```python
from build123d import *

# Parameters (mm, degrees)
SKETCH1_R               = 20
BOSS_EXTRUDE1_DEPTH     = 4
SKETCH2_R               = 1.25
CUT_EXTRUDE1_DEPTH      = 29.565713714
CAVITY1_START           = 2.8
CAVITY1_OUTLINE_R       = 0.675
CAVITY1_OUTLINE_R_2     = 0.6
CAVITY1_OUTLINE_R_3     = 2.5
CAVITY1_DEPTH           = 1.2
CAVITY1_START_2         = 3.4
CAVITY1_2_OUTLINE_R     = 2.5
CAVITY1_2_OUTLINE_R_2   = 1.25
CAVITY1_2_DEPTH         = 0.6
CUT_EXTRUDE2_START      = -2
CUT_EXTRUDE2_DEPTH      = 2
CUT_EXTRUDE3_START      = -1.2
CUT_EXTRUDE3_DEPTH      = 1.2
CUT_EXTRUDE4_DEPTH      = 1.2
SKETCH6_R               = 1.25
CUT_EXTRUDE5_DEPTH      = 29.565713714
CIRPATTERN1_COUNT       = 4
CUT_EXTRUDE6_DEPTH      = 29.422526278
CUT_EXTRUDE6_DEPTH_BACK = 2.4
SKETCH7_R               = 3.8
SKETCH8_R               = 20
SKETCH8_R_2             = 2.5
SKETCH8_R_3             = 1.25
BOSS_EXTRUDE2_DEPTH     = 3.5
CUT_EXTRUDE7_DEPTH      = 2.5
SKETCH10_R              = 2.5
SKETCH10_R_2            = 1.25
BOSS_EXTRUDE4_DEPTH     = 0.8
SKETCH11_R              = 2.5
SKETCH11_R_2            = 1.25
BOSS_EXTRUDE5_DEPTH     = 1.2
SKETCH12_R              = 3.8
CUT_EXTRUDE8_DEPTH      = 0.8


# Read off the part's stored shape, not the designer's step: Cavity1
with BuildPart() as part:
    # Sketch1 → Boss-Extrude1 (new body)
    with BuildSketch(Plane.XY):
        Circle(SKETCH1_R)
    extrude(amount=BOSS_EXTRUDE1_DEPTH)

    # Sketch2 → Cut-Extrude1 (cut, through all)
    with BuildSketch(Plane.XY.offset(4)):
        Circle(SKETCH2_R)
    extrude(amount=-CUT_EXTRUDE1_DEPTH, mode=Mode.SUBTRACT)

    # Cavity1 outline → Cavity1 (cut)
    with BuildSketch(Plane.XY.offset(CAVITY1_START)):
        with BuildLine():
            ThreePointArc((2.993325909, 2), (2.762479071, 2.308399745), (2.5, 2.590366769))
            Line((2.5, 2.590366769), (2.5, 3.6))
            Line((2.5, 3.6), (2, 15.6))
            ThreePointArc((2, 15.6), (0, 17.6), (-2, 15.6))
            Line((-2, 15.6), (-2.5, 3.6))
            Line((-2.5, 3.6), (-2.5, 2.590366769))
            ThreePointArc((-2.5, 2.590366769), (-2.762479071, 2.308399745), (-2.993325909, 2))
            Line((-2.993325909, 2), (-6.6, 2))
            ThreePointArc((-6.6, 2), (-8.6, 0), (-6.6, -2))
            Line((-6.6, -2), (-2.993325909, -2))
            ThreePointArc((-2.993325909, -2), (-2.762479071, -2.308399745), (-2.5, -2.590366769))
            Line((-2.5, -2.590366769), (-2.5, -3.6))
            Line((-2.5, -3.6), (-2, -15.6))
            ThreePointArc((-2, -15.6), (0, -17.6), (2, -15.6))
            Line((2, -15.6), (2.5, -3.6))
            Line((2.5, -3.6), (2.5, -2.590366769))
            ThreePointArc((2.5, -2.590366769), (2.762479071, -2.308399745), (2.993325909, -2))
            Line((2.993325909, -2), (6.6, -2))
            ThreePointArc((6.6, -2), (8.6, 0), (6.6, 2))
            Line((6.6, 2), (2.993325909, 2))
        make_face()
        with Locations((0, -15.6)):
            Circle(CAVITY1_OUTLINE_R, mode=Mode.SUBTRACT)
        with Locations((0, -13.4)):
            Circle(CAVITY1_OUTLINE_R, mode=Mode.SUBTRACT)
        with Locations((0, -11.2)):
            Circle(CAVITY1_OUTLINE_R, mode=Mode.SUBTRACT)
        with Locations((0, -9)):
            Circle(CAVITY1_OUTLINE_R, mode=Mode.SUBTRACT)
        with Locations((0, -6.8)):
            Circle(CAVITY1_OUTLINE_R, mode=Mode.SUBTRACT)
        with Locations((0, -4.6)):
            Circle(CAVITY1_OUTLINE_R, mode=Mode.SUBTRACT)
        with Locations((-6.6, 0)):
            Circle(CAVITY1_OUTLINE_R_2, mode=Mode.SUBTRACT)
        with Locations((-4.6, 0)):
            Circle(CAVITY1_OUTLINE_R_2, mode=Mode.SUBTRACT)
        Circle(CAVITY1_OUTLINE_R_3, mode=Mode.SUBTRACT)
        with Locations((0, 4.6)):
            Circle(CAVITY1_OUTLINE_R, mode=Mode.SUBTRACT)
        with Locations((0, 6.8)):
            Circle(CAVITY1_OUTLINE_R, mode=Mode.SUBTRACT)
        with Locations((4.6, 0)):
            Circle(CAVITY1_OUTLINE_R_2, mode=Mode.SUBTRACT)
        with Locations((6.6, 0)):
            Circle(CAVITY1_OUTLINE_R_2, mode=Mode.SUBTRACT)
        with Locations((0, 9)):
            Circle(CAVITY1_OUTLINE_R, mode=Mode.SUBTRACT)
        with Locations((0, 11.2)):
            Circle(CAVITY1_OUTLINE_R, mode=Mode.SUBTRACT)
        with Locations((0, 13.4)):
            Circle(CAVITY1_OUTLINE_R, mode=Mode.SUBTRACT)
        with Locations((0, 15.6)):
            Circle(CAVITY1_OUTLINE_R, mode=Mode.SUBTRACT)
    extrude(amount=CAVITY1_DEPTH, mode=Mode.SUBTRACT)

    # Cavity1 2 outline → Cavity1 2 (cut)
    with BuildSketch(Plane.XY.offset(CAVITY1_START_2)):
        Circle(CAVITY1_2_OUTLINE_R)
        Circle(CAVITY1_2_OUTLINE_R_2, mode=Mode.SUBTRACT)
    extrude(amount=CAVITY1_2_DEPTH, mode=Mode.SUBTRACT)

    # Sketch3 → Cut-Extrude2 (cut)
    with BuildSketch(Plane.XY.offset(3.4).offset(CUT_EXTRUDE2_START)):
        with BuildLine():
            ThreePointArc((-2.5, 0), (0, -2.5), (2.5, 0))
            ThreePointArc((2.5, 0), (0, 2.5), (-2.5, 0))
        make_face()
    extrude(amount=CUT_EXTRUDE2_DEPTH, mode=Mode.SUBTRACT)

    # Sketch4 → Cut-Extrude3 (cut)
    with BuildSketch(Plane.XY.offset(4).offset(CUT_EXTRUDE3_START)):
        with BuildLine():
            Line((-6.6, -2), (-2.993325909, -2))
            ThreePointArc((-2.993325909, -2), (-2.762479071, -2.308399745), (-2.5, -2.590366769))
            Line((-2.5, -2.590366769), (-2.5, -3.6))
            Line((-2.5, -3.6), (-2, -15.6))
            ThreePointArc((-2, -15.6), (0, -17.6), (2, -15.6))
            Line((2, -15.6), (2.5, -3.6))
            Line((2.5, -3.6), (2.5, -2.590366769))
            ThreePointArc((2.5, -2.590366769), (2.762479071, -2.308399745), (2.993325909, -2))
            Line((2.993325909, -2), (6.6, -2))
            ThreePointArc((6.6, -2), (8.6, 0), (6.6, 2))
            Line((6.6, 2), (2.993325909, 2))
            ThreePointArc((2.993325909, 2), (2.762479071, 2.308399745), (2.5, 2.590366769))
            Line((2.5, 2.590366769), (2.5, 3.6))
            Line((2.5, 3.6), (2, 15.6))
            ThreePointArc((2, 15.6), (0, 17.6), (-2, 15.6))
            Line((-2, 15.6), (-2.5, 3.6))
            Line((-2.5, 3.6), (-2.5, 2.590366769))
            ThreePointArc((-2.5, 2.590366769), (-2.762479071, 2.308399745), (-2.993325909, 2))
            Line((-2.993325909, 2), (-6.6, 2))
            ThreePointArc((-6.6, 2), (-8.6, 0), (-6.6, -2))
        make_face()
    extrude(amount=CUT_EXTRUDE3_DEPTH, mode=Mode.SUBTRACT)

    # Sketch5 → Cut-Extrude4 (cut)
    with BuildSketch(Plane.XY.offset(4)):
        with BuildLine():
            Line((-6.6, -2.03), (-3.00931886, -2.03))
            ThreePointArc((-3.00931886, -2.03), (-2.784441978, -2.328901645), (-2.53, -2.603075105))
            Line((-2.53, -2.603075105), (-2.53, -3.600624729))
            Line((-2.53, -3.600624729), (-2.029999903, -15.600627053))
            ThreePointArc((-2.029999903, -15.600627053), (0, -17.63), (2.029999903, -15.600627053))
            Line((2.029999903, -15.600627053), (2.53, -3.600624729))
            Line((2.53, -3.600624729), (2.53, -2.603075105))
            ThreePointArc((2.53, -2.603075105), (2.784441978, -2.328901645), (3.00931886, -2.03))
            Line((3.00931886, -2.03), (6.6, -2.03))
            ThreePointArc((6.6, -2.03), (8.63, 0), (6.6, 2.03))
            Line((6.6, 2.03), (3.00931886, 2.03))
            ThreePointArc((3.00931886, 2.03), (2.784441978, 2.328901645), (2.53, 2.603075105))
            Line((2.53, 2.603075105), (2.53, 3.600624729))
            Line((2.53, 3.600624729), (2.029999903, 15.600627053))
            ThreePointArc((2.029999903, 15.600627053), (0, 17.63), (-2.029999903, 15.600627053))
            Line((-2.029999903, 15.600627053), (-2.53, 3.600624729))
            Line((-2.53, 3.600624729), (-2.53, 2.603075105))
            ThreePointArc((-2.53, 2.603075105), (-2.784441978, 2.328901645), (-3.00931886, 2.03))
            Line((-3.00931886, 2.03), (-6.6, 2.03))
            ThreePointArc((-6.6, 2.03), (-8.63, 0), (-6.6, -2.03))
        make_face()
    extrude(amount=-CUT_EXTRUDE4_DEPTH, mode=Mode.SUBTRACT)

    # Sketch6 → Cut-Extrude5 (cut, through all)
    with BuildSketch(Plane.XY.offset(4)):
        with Locations((5.303300859, 5.303300859)):
            Circle(SKETCH6_R)
        with Locations((8.838834765, 8.838834765)):
            Circle(SKETCH6_R)
        with Locations((12.374368671, 12.374368671)):
            Circle(SKETCH6_R)
    cut_extrude5 = extrude(amount=-CUT_EXTRUDE5_DEPTH, mode=Mode.SUBTRACT)

    # CirPattern1: Cut-Extrude5 ×4 about axis
    cirpattern1_axis = Axis((0, 0, 0), (0, 0, 1))
    for i in range(1, CIRPATTERN1_COUNT):
        add(cut_extrude5.rotate(cirpattern1_axis, i * 360 / CIRPATTERN1_COUNT), mode=Mode.SUBTRACT)

    # Sketch7 → Cut-Extrude6 (cut, two sides: drawn at the far end of the back side and taken through both)
    with BuildSketch(Plane.XY.offset(2.8).offset(-CUT_EXTRUDE6_DEPTH_BACK)):
        with Locations(Location((0, 0, 0), (0, 0, 147.709612918))):
            Circle(SKETCH7_R)
    extrude(amount=CUT_EXTRUDE6_DEPTH + CUT_EXTRUDE6_DEPTH_BACK, mode=Mode.SUBTRACT)

    # Sketch8 → Boss-Extrude2 (add)
    with BuildSketch(Plane(origin=(0, 0, 0), x_dir=(-1, 0, 0), z_dir=(0, 0, -1))):
        Circle(SKETCH8_R)
        Circle(SKETCH8_R_2, mode=Mode.SUBTRACT)
        with Locations(Location((12.374368671, 12.374368671, 0), (0, 0, 90))):
            Circle(SKETCH8_R_3, mode=Mode.SUBTRACT)
        with Locations(Location((-12.374368671, 12.374368671, 0), (0, 0, 180))):
            Circle(SKETCH8_R_3, mode=Mode.SUBTRACT)
        with Locations(Location((-8.838834765, 8.838834765, 0), (0, 0, 180))):
            Circle(SKETCH8_R_3, mode=Mode.SUBTRACT)
        with Locations(Location((-5.303300859, 5.303300859, 0), (0, 0, 180))):
            Circle(SKETCH8_R_3, mode=Mode.SUBTRACT)
        with Locations((12.374368671, -12.374368671)):
            Circle(SKETCH8_R_3, mode=Mode.SUBTRACT)
        with Locations((8.838834765, -8.838834765)):
            Circle(SKETCH8_R_3, mode=Mode.SUBTRACT)
        with Locations((5.303300859, -5.303300859)):
            Circle(SKETCH8_R_3, mode=Mode.SUBTRACT)
        with Locations(Location((-12.374368671, -12.374368671, 0), (0, 0, 270))):
            Circle(SKETCH8_R_3, mode=Mode.SUBTRACT)
        with Locations(Location((-8.838834765, -8.838834765, 0), (0, 0, 270))):
            Circle(SKETCH8_R_3, mode=Mode.SUBTRACT)
        with Locations(Location((-5.303300859, -5.303300859, 0), (0, 0, 270))):
            Circle(SKETCH8_R_3, mode=Mode.SUBTRACT)
        with Locations(Location((5.303300859, 5.303300859, 0), (0, 0, 90))):
            Circle(SKETCH8_R_3, mode=Mode.SUBTRACT)
        with Locations(Location((8.838834765, 8.838834765, 0), (0, 0, 90))):
            Circle(SKETCH8_R_3, mode=Mode.SUBTRACT)
    extrude(amount=BOSS_EXTRUDE2_DEPTH)

    # Sketch9 → Cut-Extrude7 (cut)
    with BuildSketch(Plane.XY.offset(4)):
        with BuildLine():
            Line((2.58, 3.601665944), (2.07999932, 15.601682271))
            ThreePointArc((2.07999932, 15.601682271), (0, 17.68), (-2.07999932, 15.601682271))
            Line((-2.07999932, 15.601682271), (-2.58, 3.601665944))
            Line((-2.58, 3.601665944), (-2.58, 2.857638886))
            ThreePointArc((-2.58, 2.857638886), (-2.935746402, 2.490761543), (-3.23976851, 2.08))
            Line((-3.23976851, 2.08), (-6.6, 2.08))
            ThreePointArc((-6.6, 2.08), (-8.68, 0), (-6.6, -2.08))
            Line((-6.6, -2.08), (-3.23976851, -2.08))
            ThreePointArc((-3.23976851, -2.08), (-2.935746402, -2.490761543), (-2.58, -2.857638886))
            Line((-2.58, -2.857638886), (-2.58, -3.601665944))
            Line((-2.58, -3.601665944), (-2.07999932, -15.601682271))
            ThreePointArc((-2.07999932, -15.601682271), (0, -17.68), (2.07999932, -15.601682271))
            Line((2.07999932, -15.601682271), (2.58, -3.601665944))
            Line((2.58, -3.601665944), (2.58, -2.857638886))
            ThreePointArc((2.58, -2.857638886), (2.935746402, -2.490761543), (3.23976851, -2.08))
            Line((3.23976851, -2.08), (6.6, -2.08))
            ThreePointArc((6.6, -2.08), (8.68, 0), (6.6, 2.08))
            Line((6.6, 2.08), (3.23976851, 2.08))
            ThreePointArc((3.23976851, 2.08), (2.935746402, 2.490761543), (2.58, 2.857638886))
            Line((2.58, 2.857638886), (2.58, 3.601665944))
        make_face()
    extrude(amount=-CUT_EXTRUDE7_DEPTH, mode=Mode.SUBTRACT)

    # Sketch10 → Boss-Extrude4 (add)
    with BuildSketch(Plane(origin=(0, 0, 0), x_dir=(-1, 0, 0), z_dir=(0, 0, -1))):
        Circle(SKETCH10_R)
        with Locations(Location((0, 0, 0), (0, 0, 180))):
            Circle(SKETCH10_R_2, mode=Mode.SUBTRACT)
    extrude(amount=BOSS_EXTRUDE4_DEPTH)

    # Sketch11 → Boss-Extrude5 (add)
    with BuildSketch(Plane(origin=(0, 0, -0.8), x_dir=(-1, 0, 0), z_dir=(0, 0, -1))):
        Circle(SKETCH11_R)
        with Locations(Location((0, 0, 0), (0, 0, 180))):
            Circle(SKETCH11_R_2, mode=Mode.SUBTRACT)
    extrude(amount=BOSS_EXTRUDE5_DEPTH)

    # Sketch12 → Cut-Extrude8 (cut)
    with BuildSketch(Plane.XY.offset(0.4)):
        Circle(SKETCH12_R)
    extrude(amount=-CUT_EXTRUDE8_DEPTH, mode=Mode.SUBTRACT)


solid = part.part
```
Work out the finished part from the listing and answer in its coordinate system (mm). A direction names the side the tool comes from. Round coordinates to 2 decimals unless told otherwise and drop trailing zeros. Loops run counter-clockwise (first coordinate to the right, second up) from the corner with the lowest first, then second, coordinate; pieces in that order, holes last. Notation, with made-up numbers: M 69.25,12 L 84.25,12 A30 cw 84.25,39 Z; hole C 46,16.5 d5. An arc over 180 degrees is marked long. One line per question, with ' | ' between items.
Q1. Each of these flat-tipped pins is pushed along its axis until it touches: pin 1 Ø1.5 at (x, y) = (5.3, 5.3) entering from -Z; pin 2 Ø0.6 at (y, z) = (3.5, 2.5) entering from +X; pin 3 Ø4 at (y, z) = (8, -2.5) entering from +X; pin 4 Ø3 at (x, y) = (-8.84, 8.84) entering from -Z. Where does it stop, or does it pass through?
Conclusion:
pin 1: passes through | pin 2: stops at x = 19.74 | pin 3: stops at x = 19.08 | pin 4: stops at z = -3.5
Q2. Find section B-B, the plane y = 9.5. Give the vertices of the cut face in (x, z), then the cut area to 4 significant figures.
Conclusion:
outline: M -17.6,-3.5 L -9.9,-3.5 L -9.9,4 L -17.6,4 Z; M -7.78,-3.5 L 7.78,-3.5 L 7.78,4 L 2.33,4 L 2.33,1.5 L -2.33,1.5 L -2.33,4 L -7.78,4 Z; M 9.9,-3.5 L 17.6,-3.5 L 17.6,4 L 9.9,4 Z | area: 220.5 mm2
Q3. The mould has two halves that part along X. Classify faces 4 (the flat face through (4, -4, 4)), 5 (the flat face through (-2.326, 9.686, 2.768)): +X half, -X half, draft (parallel to the pull), parting line (faces both ways), or undercut.
Conclusion:
face 4: draft | face 5: undercut
Q4. Consider line 1 along X through (y, z) = (13.5, 2.25); line 2 along Y through (x, z) = (-12, -1.5); line 3 along Y through (x, z) = (-5, -0.25). Determine where each line is inside the solid, lowest interval first. Write a range as from..to.
Conclusion:
line 1: x = -14.76..-12.92, -11.83..-2.17, 2.17..11.83, 12.92..14.76 | line 2: y = -16..-13.57, -11.18..11.18, 13.57..16 | line 3: y = -19.36..-6.52, -4.09..4.09, 6.52..19.36
Q5. Find section C-C, the plane z = 2. State how many separate pieces and enclosed holes the cut face has, then the cut area to 3 significant figures.
Conclusion:
separate pieces: 1 | enclosed holes: 13 | area: 987 mm2
Q6. A tool of negligible diameter and unlimited length cuts with its end or side. For faces 1 (the flat face through (0, -4, -3.5)), 2 (the cylindrical face through (8.68, -0.05, 2.77)), 3 (the flat face through (1, -1, -2)), from which of +Z, -Z, +X, -X, +Y, -Y can it reach the whole face along a straight path? Write none if from no direction.
Conclusion:
face 1: -Z, +X, -X, +Y, -Y | face 2: +Z | face 3: -Z
Q7. Find section A-A, the plane x = 0. Give the vertices of the cut face in (y, z).
Conclusion:
outline: M -20,-3.5 L -2.5,-3.5 L -2.5,-2 L -1.25,-2 L -1.25,-0.4 L -3.8,-0.4 L -3.8,1.5 L -17.68,1.5 L -17.68,4 L -20,4 Z; M 1.25,-2 L 2.5,-2 L 2.5,-3.5 L 20,-3.5 L 20,4 L 17.68,4 L 17.68,1.5 L 3.8,1.5 L 3.8,-0.4 L 1.25,-0.4 Z
